The listing builds one solid part. Answer for the finished solid, in the listing's coordinates (mm). Coordinates: 2 decimals unless noted, no trailing zeros. Order: outer loops, then holes, each group sorted by start corner. A loop starts at its lowest first (then second) coordinate and runs counter-clockwise, first axis right, second up.
Autodesk Fusion 360 part; units mm, degrees
sketch "Sketch1" plane through (0, 0, 0) normal (0, 0, 1) x (1, 0, 0)
  line L0 (25, 0) -> (25, 8.5)
  line L1 (25, 8.5) -> (0, 8.5)
  line L2 (0, 8.5) -> (0, 0)
  arc A0 (19, 0) -> (6, 0) centre (12.5, 0) ccw
  line L3 (0, 0) -> (6, 0)
  line L4 (19, 0) -> (25, 0)
  dimension "d1" = 25
  dimension "d2" = 8.5
  dimension "d3" = 13
extrude "Extrude1" add sketch "Sketch1" along normal blind 5
sketch "Sketch2" plane through (0, 8.5, 0) normal (0, 1, 0) x (-1, 0, 0)
  line L0 (-25, 0) -> (0, 0)
  line L1 (0, 0) -> (0, 5)
  line L2 (0, 5) -> (-25, 5)
  line L3 (-25, 5) -> (-25, 0)
  line L4 (-19, 0) -> (-19, 5)
  line L5 (-6, 0) -> (-6, 5)
  line L6 (0, 5) -> (-6, 0) construction
  line L7 (-12.5, 0) -> (-12.5, 5)
  circle A0 centre (-3, 2.5) radius 1
  circle A1 centre (-22, 2.5) radius 1
  dimension "d6" = 2
extrude "Extrude2" cut sketch "Sketch2" against normal through all contours A0 | A1
fillet "Fillet1" radius 0.2 6 edges at (0, 0, 2.5) (3, 0, 0) (3, 0, 5) (22, 0, 5) (25, 0, 2.5) (22, 0, 0)
1) Section D-D (y = 7) is taken. Give the vertices of the cut face in (x, z).
2) Section A-A (y = 6) is taken. Give the vertices of the cut face in (x, z), then the cut area to 3 significant figures.
3) Section B-B (x = 22) is taken. Give the vertices of the cut face in (y, z).
4) Determine the mould class of faces 1 (the face through (23, 4.3, 2.5)), 2 (the face through (25, 4, 2)), 3 (the face through (4, 4.3, 2.5)), 4 (the face through (12, 7, 0)) for opening direction X: released by +X, released by -X, zero draft, split by the parting line, or undercut.
5) Section C-C (z = 2.5) is taken. Give the vertices of the cut face in (x, y), then the cut area to 3 significant figures.
6) Each of these flat-tipped pins is pushed along its axis until it touches: P1, Ø2, axis at x = 9, z = 2, coming from the -Y side; P2, Ø1.5, axis at x = 13, z = 1, coming from the -Y side. Where does it stop, or does it pass through?
7) Consider L1, parallel to Z at x = 22, y = 2.25; L2, parallel to X at y = 2.25, z = 1.7; L3, parallel to X at y = 1.5, z = 2.35. Determine where each line is inside the solid, lowest interval first.
Filled sheet:
1. outline: (0, 0) - (25, 0) - (25, 5) - (0, 5) - close; hole circle Ø2 at (3, 2.5); hole circle Ø2 at (22, 2.5)
2. outline: (0, 0) - (10, 0) - (10, 5) - (0, 5) - close; (15, 0) - (25, 0) - (25, 5) - (15, 5) - close; hole circle Ø2 at (3, 2.5); hole circle Ø2 at (22, 2.5)
2. area: 93.7 mm2
3. outline: (0, 0.2) arc R0.2 ccw to (0.2, 0) - (8.5, 0) - (8.5, 1.5) - (0, 1.5) - close; (0, 3.5) - (8.5, 3.5) - (8.5, 5) - (0.2, 5) arc R0.2 ccw to (0, 4.8) - close
4. face 1: undercut
4. face 2: released by +X
4. face 3: undercut
4. face 4: zero draft
5. outline: (0, 0.2) arc R0.2 ccw to (0.2, 0) - (2, 0) - (2, 8.5) - (0, 8.5) - close; (4, 0) - (6, 0) arc R6.5 cw to (19, 0) - (21, 0) - (21, 8.5) - (4, 8.5) - close; (23, 0) - (24.8, 0) arc R0.2 ccw to (25, 0.2) - (25, 8.5) - (23, 8.5) - close
5. area: 112 mm2
6. P1: stops at y = 4.69
6. P2: stops at y = 6.38
7. L1: z = 0 to 1.5, 3.5 to 5
7. L2: x = 0 to 2.4, 3.6 to 6.4, 18.6 to 21.4, 22.6 to 25
7. L3: x = 0 to 2.01, 3.99 to 6.18, 18.82 to 21.01, 22.99 to 25
